from build123d import *

# Parameters (mm, degrees)
F0_W      = 11
F0_H      = 42
F1_DEPTH  = 10
F2_T      = 2
F3_W      = 15
F3_H      = 20
F4_DEPTH  = 2
F6_DEPTH  = 2
F8_R      = 1.25
F9_DEPTH  = 2.001
F10_R     = 1.25
F11_DEPTH = 15.001
F12_R     = 2


# Not quite as in the source:
# - a pattern or mirror of a feature is missing from the dataset's text; its kind, count and spacing are read off the source's solid


with BuildPart() as f1:
    # F0 (on Top) → F1 (new body)
    with BuildSketch(Plane.XY):
        with Locations((5.5, 21)):
            Rectangle(F0_W, F0_H)
    extrude(amount=F1_DEPTH)

    # F2
    f2_openings = [f1.faces().sort_by_distance(p)[0] for p in [
        (5.5, 21, 10),
        (5.5, 21, 0),
    ]]
    offset(amount=F2_T, openings=f2_openings, kind=Kind.INTERSECTION)

    # F3 (on Top) → F4 (join)
    with BuildSketch(Plane.XY):
        with Locations((5.5, -12)):
            Rectangle(F3_W, F3_H)
    extrude(amount=F4_DEPTH)

    # F5 (on face) → F6 (join)
    with BuildSketch(Plane.YZ.offset(13)):
        Polygon((-2, 10), (-22, 2), (-2, 2), align=None)
    f6 = extrude(amount=-F6_DEPTH)

    # F6_copies: F6 across plane
    add(f6.mirror(Plane(origin=(5.5, 0, 0), x_dir=(0, 0, -1), z_dir=(-1, 0, 0))))

    # F8 (on face) → F9 (cut, through all)
    with BuildSketch(Plane.XY.offset(2)):
        with Locations((5.5, -14)):
            Circle(F8_R)
    extrude(amount=-F9_DEPTH, mode=Mode.SUBTRACT)

    # F10 (on face) → F11 (cut, through all)
    with BuildSketch(Plane.YZ.offset(13)):
        with Locations((11, 5)):
            Circle(F10_R)
        with Locations((31, 5)):
            Circle(F10_R)
    extrude(amount=-F11_DEPTH, mode=Mode.SUBTRACT)

    # F12
    f12_edges = [f1.edges().sort_by_distance(p)[0] for p in [
        (-2, -22, 1),
        (13, -22, 1),
        (13, 44, 5),
        (-2, 44, 5),
    ]]
    fillet(f12_edges, radius=F12_R)


solid = f1.part
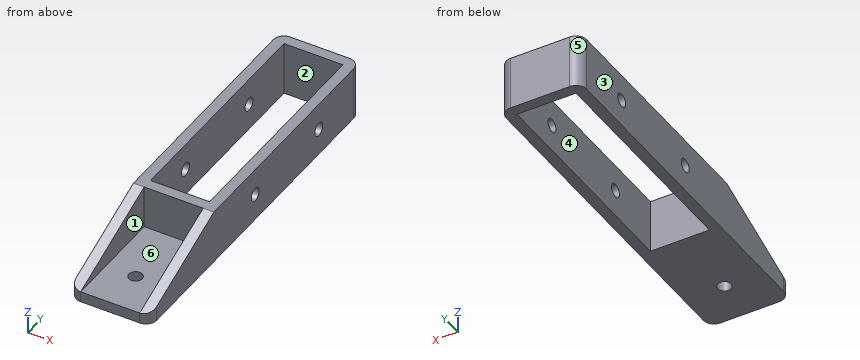
Source: CAD feature listing. Evaluate the final solid. Frame: model axes, mm. Face numbers are marked on the shaded views. A direction names the side the tool comes from. Give positions to 0.01 mm unless a question says otherwise; leave off trailing zeros. Order: outer loops, then holes, each group sorted by start corner. A loop starts at its lowest first (then second) coordinate and runs counter-clockwise, first axis right, second up. Notation, with made-up numbers: (76, 36.5) -> (129, 36.5) arc R21 cw to (129, 49.5) -> close; hole circle Ø9 at (82.25, 25.25). An arc over 180 degrees is marked (long way). Use a Markdown table: item, result.
1) Section query A-A, the plane y = 11. Return the cut outline in (x, z).
Answer list:
| item | result |
|---|---|
| outline | (-2, 0) -> (0, 0) -> (0, 3.75) -> (-2, 3.75) -> close; (-2, 6.25) -> (0, 6.25) -> (0, 10) -> (-2, 10) -> close; (11, 0) -> (13, 0) -> (13, 3.75) -> (11, 3.75) -> close; (11, 6.25) -> (13, 6.25) -> (13, 10) -> (11, 10) -> close |
2) Ray query, line 1 along X through (y, z) = (0.5, 8.5); line 2 along Y through (x, z) = (0.5, 9); line 3 along Y through (x, z) = (6.5, 1.75). Return the intervals inside material, ascending. Write a range as [from, to].
Answer list:
| item | result |
|---|---|
| line 1 | [-2, 0], [11, 13] |
| line 2 | [-2, 0], [42, 44] |
| line 3 | [-22, -14.75], [-13.25, 0], [42, 44] |
3) Section query D-D, the plane y = 35.5. Return the cut outline in (x, z).
Answer list:
| item | result |
|---|---|
| outline | (-2, 0) -> (0, 0) -> (0, 10) -> (-2, 10) -> close; (11, 0) -> (13, 0) -> (13, 10) -> (11, 10) -> close |
4) Mould query, pull axis Y, two halves, no side actions, for the marked faces 4, 5 and 6. Classes: +Y half, -Y half, draft (parallel to the pull), parting line (faces both ways), or undercut.
Answer list:
| item | result |
|---|---|
| face 4 | undercut |
| face 5 | +Y half |
| face 6 | draft |
5) Contact query for flat-ended pins moving along their axis: P1, Ø5, axis at x = 6.5, z = 3.5, coming from the -Y side; P2, Ø4, axis at x = 6, z = 7, coming from the -Y side; P3, Ø2, axis at y = 11, z = 5, coming from the -X side; P4, Ø4, axis at x = 5.5, y = -14, coming from the +Z side. Output: stop coordinate, or through.
Answer list:
| item | result |
|---|---|
| P1 | y = -22 |
| P2 | y = -2 |
| P3 | through |
| P4 | z = 2 |
6) Reachability of the marked faces 1, 2 and 3 from +Z, -Z, +X, -X, +Y, -Y: full face, straight path, thin tool, end or side. Return the list, or none.
Answer list:
| item | result |
|---|---|
| face 1 | +Z, -Y |
| face 2 | +Z, -Z |
| face 3 | +Z, -Z, -X, +Y, -Y |
7) Section query C-C, the plane z = 5. Count the separate pieces of the cut face and the enclosed holes in it, then the cut area to 3 significant figures.
Answer list:
| item | result |
|---|---|
| separate pieces | 4 |
| enclosed holes | 0 |
| area | 256 mm² |
8) Section query B-B, the plane x = 5.5. Return the cut outline in (y, z), then the cut area to 3 significant figures.
Answer list:
| item | result |
|---|---|
| outline | (-22, 0) -> (-15.25, 0) -> (-15.25, 2) -> (-22, 2) -> close; (-12.75, 0) -> (0, 0) -> (0, 10) -> (-2, 10) -> (-2, 2) -> (-12.75, 2) -> close; (42, 0) -> (44, 0) -> (44, 10) -> (42, 10) -> close |
| area | 75.0 mm² |
